Verification items for the finished model (mm, model axes). A direction names the side the tool comes from. Round coordinates to 2 decimals unless told otherwise and drop trailing zeros. Order: outer loops, then holes, each group sorted by start corner. A loop starts at its lowest first (then second) coordinate and runs counter-clockwise, first axis right, second up. Notation, with made-up numbers: (17.25, -0.75) -> (53.25, -0.75) arc R29 cw to (53.25, 36.25) -> close; hole circle Ø1 at (-4.5, 18). An arc over 180 degrees is marked (long way). Return JSON: item names as keys, results as strings. Group by question number.
Item 1: Draft check along X on faces 1 (the flat face through (107, -5, -120.752)), 2 (the flat face through (81.27, 2, -105)), 3 (the flat face through (163, 2, -143.252)), 4 (the flat face through (165.12, 2, -131)). Enter one of: pulls with the +X half, pulls with the -X half, needs draft (parallel to the pull), parting line crosses it, or undercut.
Item 2: Sectioned sample at A-A on z = -137. Record the cut outline in (x, y), plus the area to 3 significant figures.
Item 3: Sectioned sample at B-B on y = 2. Record the cut outline in (x, z), plus the area to 3 significant figures.
Item 4: Sectioned sample at D-D on y = -7.75. Record the cut outline in (x, z), plus the area to 3 significant figures.
Item 5: Access from +Z, -Z, +X, -X, +Y, -Y to the whole of each face (thin tool, end or side, straight path). Record for faces 5 (the flat face through (160.12, 2, -131)), 6 (the flat face through (109.07, 9, -131)), 7 (the flat face through (107, -5, -140.752)).
Item 6: Scan lines: probe 1 along Y at (x, z) = (274, -101); probe 2 along Z at (x, y) = (199.5, 1.75); probe 3 along X at (y, z) = (7.25, -128.5). Record each from-to range of solid material in increasing order. Write a range as from..to.
Item 7: Depth check by flat-ended pin: pin 1 Ø1.2 at (x, y) = (106.5, -3) entering from -Z; pin 2 Ø5 at (y, z) = (10.5, -135.5) entering from -X; pin 3 Ø1.2 at (x, y) = (106.5, -4.5) entering from +Z. Enter the tip coordinate at first touch or a pass-through.
Item 8: Sectioned sample at C-C on x = 212.5. Record the cut outline in (y, z), plus the area to 3 significant figures.
```python
from build123d import *

# Parameters (mm, degrees)
BOSS_EXTRUDE7_DEPTH      = 4
SKETCH3_W                = 34
SKETCH3_H                = 22
CUT_EXTRUDE2_DEPTH       = 4
CUT_EXTRUDE3_DEPTH       = 4
SKETCH7_W                = 4
SKETCH7_H                = 20
BOSS_EXTRUDE9_DEPTH      = 10
BOSS_EXTRUDE9_DEPTH_BACK = 14
SKETCH9_W                = 5
SKETCH9_H                = 25
CUT_EXTRUDE4_DEPTH       = 4


with BuildPart() as part:
    # Sketch1 → Boss-Extrude7 (new body)
    with BuildSketch(Plane(origin=(0, 0, 0), x_dir=(1, 0, 0), z_dir=(0, 1, 0))):
        with BuildLine():
            Line((101.270150391, 181.252283774), (275.970150391, 181.252283774))
            ThreePointArc((275.970150391, 181.252283774), (290.112286015, 175.394419397), (295.970150391, 161.252283774))
            Line((295.970150391, 161.252283774), (295.970150391, 100.252283774))
            ThreePointArc((295.970150391, 100.252283774), (290.112286015, 86.11014815), (275.970150391, 80.252283774))
            Line((275.970150391, 80.252283774), (101.270150391, 80.252283774))
            ThreePointArc((101.270150391, 80.252283774), (87.128014768, 86.11014815), (81.270150391, 100.252283774))
            Line((81.270150391, 100.252283774), (81.270150391, 161.252283774))
            ThreePointArc((81.270150391, 161.252283774), (87.128014768, 175.394419397), (101.270150391, 181.252283774))
        make_face()
    extrude(amount=BOSS_EXTRUDE7_DEPTH)

    # Sketch3 → Cut-Extrude2 (cut)
    with BuildSketch(Plane(origin=(0, 4, 0), x_dir=(1, 0, 0), z_dir=(0, 1, 0))):
        with Locations((188.620150391, 130.752283774)):
            Rectangle(SKETCH3_W, SKETCH3_H)
    extrude(amount=-CUT_EXTRUDE2_DEPTH, mode=Mode.SUBTRACT)

    # Sketch6 → Cut-Extrude3 (cut)
    with BuildSketch(Plane(origin=(0, 4, 0), x_dir=(1, 0, 0), z_dir=(0, 1, 0))):
        Polygon((81.270150391, 151.752283774), (81.270150391, 109.752283774), (99.770150391, 120.752283774), (99.770150391, 140.752283774), align=None)
    extrude(amount=-CUT_EXTRUDE3_DEPTH, mode=Mode.SUBTRACT)

    # Sketch7 → Boss-Extrude9 (add, two sides)
    with BuildSketch(Plane(origin=(0, 4, 0), x_dir=(1, 0, 0), z_dir=(0, 1, 0))) as boss_extrude9_sk:
        with Locations((107.070150391, 130.752283774)):
            Rectangle(SKETCH7_W, SKETCH7_H)
    extrude(amount=BOSS_EXTRUDE9_DEPTH)
    extrude(boss_extrude9_sk.sketch, amount=-BOSS_EXTRUDE9_DEPTH_BACK)

    # Sketch9 → Cut-Extrude4 (cut)
    with BuildSketch(Plane(origin=(0, 0, 0), x_dir=(-1, 0, 0), z_dir=(0, -1, 0))):
        with Locations((-162.620150391, 130.752283774)):
            Rectangle(SKETCH9_W, SKETCH9_H)
    extrude(amount=-CUT_EXTRUDE4_DEPTH, mode=Mode.SUBTRACT)


solid = part.part
```
Recorded:
{
 "1": {"face 1": "needs draft", "face 2": "pulls with the -X half", "face 3": "undercut", "face 4": "undercut"},
 "2": {"outline": "(99.77, 0) -> (105.07, 0) -> (105.07, -10) -> (109.07, -10) -> (109.07, 0) -> (160.12, 0) -> (160.12, 4) -> (109.07, 4) -> (109.07, 14) -> (105.07, 14) -> (105.07, 4) -> (99.77, 4) -> close; (165.12, 0) -> (171.62, 0) -> (171.62, 4) -> (165.12, 4) -> close; (205.62, 0) -> (295.97, 0) -> (295.97, 4) -> (205.62, 4) -> close", "area": "709 mm²"},
 "3": {"outline": "(81.27, -161.25) arc R20 ccw to (101.27, -181.25) -> (275.97, -181.25) arc R20 ccw to (295.97, -161.25) -> (295.97, -100.25) arc R20 ccw to (275.97, -80.25) -> (101.27, -80.25) arc R20 ccw to (81.27, -100.25) -> (81.27, -109.75) -> (99.77, -120.75) -> (99.77, -140.75) -> (81.27, -151.75) -> close; hole (160.12, -143.25) -> (165.12, -143.25) -> (165.12, -118.25) -> (160.12, -118.25) -> close; hole (171.62, -141.75) -> (205.62, -141.75) -> (205.62, -119.75) -> (171.62, -119.75) -> close", "area": "19,900 mm²"},
 "4": {"outline": "(105.07, -140.75) -> (109.07, -140.75) -> (109.07, -120.75) -> (105.07, -120.75) -> close", "area": "80.0 mm²"},
 "5": {"face 5": "+Y, -Y", "face 6": "+Z, -Z, +X, +Y", "face 7": "-Z, +X, -X, -Y"},
 "6": {"probe 1": "0..4", "probe 2": "-181.25..-141.75, -119.75..-80.25", "probe 3": "105.07..109.07"},
 "7": {"pin 1": "z = -140.75", "pin 2": "x = 105.07", "pin 3": "z = -120.75"},
 "8": {"outline": "(0, -181.25) -> (4, -181.25) -> (4, -80.25) -> (0, -80.25) -> close", "area": "404 mm²"}
}
